Job drawing, mm, ordinate dimensions from the low corner. One solid piece. Give positions to 0.01 mm unless a question says otherwise; leave off trailing zeros. Order: outer loops, then holes, each group sorted by start corner. A loop starts at its lowest first (then second) coordinate and runs counter-clockwise, first axis right, second up. Notation, with made-up numbers: M -25,25.5 L -8,25.5 A23 ccw -8,49.5 Z; hole C 89,64.5 d10. An arc over 180 degrees is marked long. Put each result on its own line as item: value. Start each with the question number.
1) Pin check, flat tip, straight feed: pin 1 (1.5 mm diameter, centred on x = 114.5, z = 1.5, fed in from -Y). Stop position of the tip, or through.
2) Cut at A-A (y = 11.5). Write the cut outline in (x, z) (1 decimal).
3) Cut at C-C (z = 2.05). Give the number of separate pieces and of enclosed holes in the cut face, and give its area (3 significant figures).
4) Cut at B-B (x = 106). Write the cut outline in (y, z), and give its area (3 significant figures).
5) Drill centre lines: line 1 (Y direction, x = 142, z = 2.3); line 2 (X direction, y = 64.5, z = 2.3); line 3 (X direction, y = 20.5, z = 2.6) (1 decimal). Where is each one in solid material? Low to high. Write a range as [from, to].
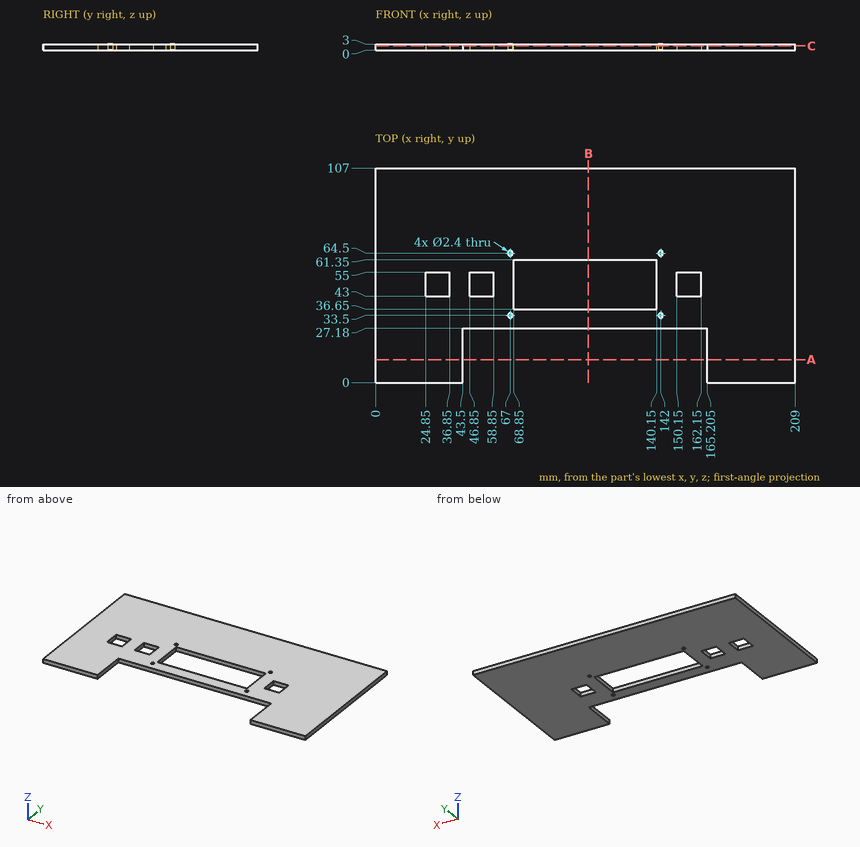
Solution:
1. pin 1: y = 27.18
2. outline: M 0,0 L 43.5,0 L 43.5,3 L 0,3 Z; M 165.2,0 L 209,0 L 209,3 L 165.2,3 Z
3. separate pieces: 1
3. enclosed holes: 8
3. area: 16,800 mm²
4. outline: M 27.18,0 L 36.65,0 L 36.65,3 L 27.18,3 Z; M 61.35,0 L 107,0 L 107,3 L 61.35,3 Z
4. area: 165 mm²
5. line 1: [27.18, 32.3], [34.7, 63.3], [65.7, 107]
5. line 2: [0, 65.8], [68.2, 140.8], [143.2, 209]
5. line 3: [0, 43.5], [165.2, 209]
